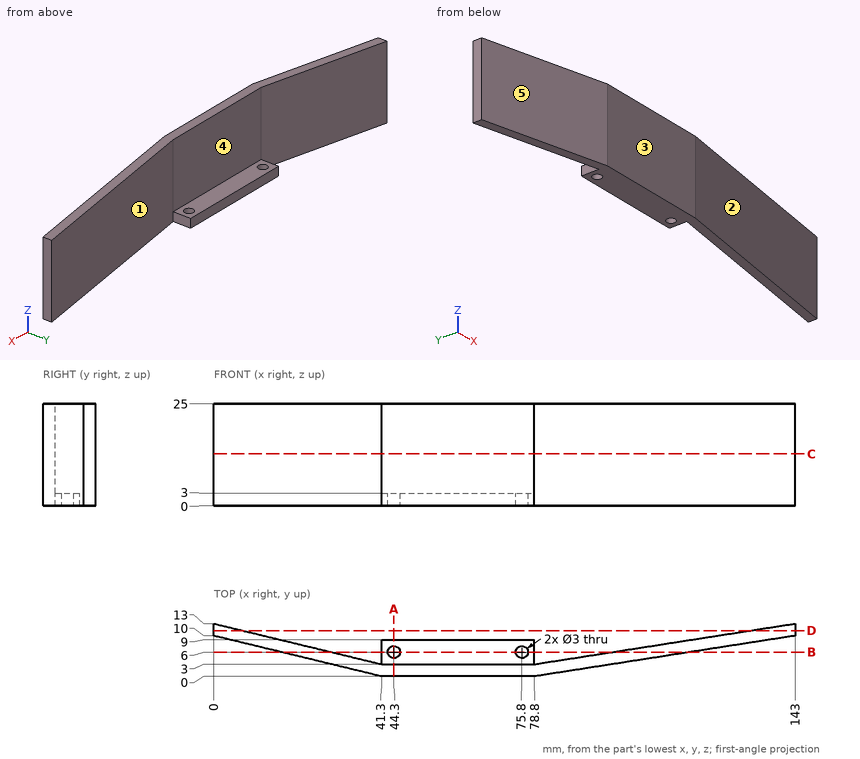
Drawing for the job (mm, zero at the part's lowest x, y, z). A direction names the side the tool comes from. Round coordinates to 2 decimals unless told otherwise and drop trailing zeros. Loops run counter-clockwise (first coordinate to the right, second up) from the corner with the lowest first, then second, coordinate; pieces in that order, holes last. Notation, with made-up numbers: (67.25, 16.25) -> (75.25, 16.25) arc R16 ccw to (75.25, 46.25) -> close; hole circle Ø7 at (73.25, -33.5). An arc over 180 degrees is marked (long way). Answer in a Markdown table with one row per item.
Item 1: Saw through at D-D (y = 11.25). Write the cut outline in (x, z) (1 decimal).
Answers below:
| item | result |
|---|---|
| outline | (0, 0) -> (7.2, 0) -> (7.2, 25) -> (0, 25) -> close; (131.8, 0) -> (143, 0) -> (143, 25) -> (131.8, 25) -> close |
Item 2: Saw through at B-B (y = 6). Write the cut outline in (x, z).
Answers below:
| item | result |
|---|---|
| outline | (16.52, 0) -> (28.91, 0) -> (28.91, 25) -> (16.52, 25) -> close; (41.3, 0) -> (42.8, 0) -> (42.8, 3) -> (41.3, 3) -> close; (45.8, 0) -> (74.3, 0) -> (74.3, 3) -> (45.8, 3) -> close; (77.3, 0) -> (78.8, 0) -> (78.8, 3) -> (77.3, 3) -> close; (98.06, 0) -> (117.32, 0) -> (117.32, 25) -> (98.06, 25) -> close |
Item 3: Saw through at A-A (x = 44.3). Write the cut outline in (y, z).
Answers below:
| item | result |
|---|---|
| outline | (0, 0) -> (4.5, 0) -> (4.5, 3) -> (3, 3) -> (3, 25) -> (0, 25) -> close; (7.5, 0) -> (9, 0) -> (9, 3) -> (7.5, 3) -> close |
Item 4: Which spindle directions (+Z, -Z, +X, -X, +Y, -Y) get a long thin tool onto all of the face, cutting with end or side? Do the marked faces 1 and 2. Say none if no direction does.
Answers below:
| item | result |
|---|---|
| face 1 | +Z, -Z, +Y |
| face 2 | +Z, -Z, +X, -Y |
Item 5: Mould opens along X. For the marked faces 3, 4 and 5 say: +X half, -X half, draft (parallel to the pull), parting line (faces both ways), or undercut.
Answers below:
| item | result |
|---|---|
| face 3 | draft |
| face 4 | undercut |
| face 5 | -X half |
Item 6: Pin check, flat tips, straight feed: pin 1 (1 mm diameter, centred on x = 96.5, z = 7.5, fed in from +Y); pin 2 (3 mm diameter, centred on x = 66, y = 6.5, fed in from +Z); pin 3 (2 mm diameter, centred on x = 18.5, z = 14, fed in from -Y). Stop position of each tip, or through.
Answers below:
| item | result |
|---|---|
| pin 1 | stops at y = 5.83 |
| pin 2 | stops at z = 3 |
| pin 3 | stops at y = 5.28 |
Item 7: Drill centre lines: L1, parallel to Y at x = 44.3, z = 1.6; L2, parallel to Y at x = 61.5, z = 2; L3, parallel to Y at x = 86, z = 8.5. Where is each one in solid material? Low to high. Write a range as [from, to].
Answers below:
| item | result |
|---|---|
| L1 | y = [0, 4.5], [7.5, 9] |
| L2 | y = [0, 9] |
| L3 | y = [1.12, 4.12] |
Item 8: Saw through at C-C (z = 12.75). Write the cut outline in (x, y), and give its area (3 significant figures).
Answers below:
| item | result |
|---|---|
| outline | (0, 10) -> (41.3, 0) -> (78.8, 0) -> (143, 10) -> (143, 13) -> (78.8, 3) -> (41.3, 3) -> (0, 13) -> close |
| area | 429 mm² |
